```python
from build123d import *

# Parameters (mm, degrees)
F0_R     = 3.5
F0_W     = 5
F0_H     = 25
F1_DEPTH = 1
F2_W     = 2
F2_H     = 12
F2_H_2   = 8
F3_DEPTH = 9.5
F4_W     = 23
F4_H     = 35
F5_DEPTH = 1


with BuildPart() as f1:
    # F0 (on Top) → F1 (new body)
    with BuildSketch(Plane.XY):
        with BuildLine():
            Line((3.5, -20), (13.5, -20))
            Line((13.5, -20), (13.5, 10))
            Line((13.5, 10), (3.5, 20))
            Line((3.5, 20), (3.5, 28.319805))
            Line((3.5, 28.319805), (26.946408, 28.319805))
            ThreePointArc((26.946408, 28.319805), (30.556224, 25.954367), (34.819805, 26.623653))
            ThreePointArc((34.819805, 26.623653), (36.975362, 27.961046), (39.041812, 29.432384))
            ThreePointArc((39.041812, 29.432384), (40.225162, 31.819805), (39.041812, 34.207227))
            ThreePointArc((39.041812, 34.207227), (36.975362, 35.678564), (34.819805, 37.015958))
            ThreePointArc((34.819805, 37.015958), (30.556224, 37.685243), (26.946408, 35.319805))
            Line((26.946408, 35.319805), (-26.946408, 35.319805))
            ThreePointArc((-26.946408, 35.319805), (-30.556224, 37.685243), (-34.819805, 37.015958))
            ThreePointArc((-34.819805, 37.015958), (-36.975362, 35.678564), (-39.041812, 34.207227))
            ThreePointArc((-39.041812, 34.207227), (-40.225162, 31.819805), (-39.041812, 29.432384))
            ThreePointArc((-39.041812, 29.432384), (-36.975362, 27.961046), (-34.819805, 26.623653))
            ThreePointArc((-34.819805, 26.623653), (-30.556224, 25.954367), (-26.946408, 28.319805))
            Line((-26.946408, 28.319805), (-3.5, 28.319805))
            Line((-3.5, 28.319805), (-3.5, 20))
            Line((-3.5, 20), (-13.5, 10))
            Line((-13.5, 10), (-13.5, -20))
            Line((-13.5, -20), (-3.5, -20))
            Line((-3.5, -20), (-3.5, -28.319805))
            Line((-3.5, -28.319805), (-26.946408, -28.319805))
            ThreePointArc((-26.946408, -28.319805), (-30.556224, -25.954367), (-34.819805, -26.623653))
            ThreePointArc((-34.819805, -26.623653), (-36.975362, -27.961046), (-39.041812, -29.432384))
            ThreePointArc((-39.041812, -29.432384), (-40.225162, -31.819805), (-39.041812, -34.207227))
            ThreePointArc((-39.041812, -34.207227), (-36.975362, -35.678564), (-34.819805, -37.015958))
            ThreePointArc((-34.819805, -37.015958), (-30.556224, -37.685243), (-26.946408, -35.319805))
            Line((-26.946408, -35.319805), (26.946408, -35.319805))
            ThreePointArc((26.946408, -35.319805), (30.556224, -37.685243), (34.819805, -37.015958))
            ThreePointArc((34.819805, -37.015958), (36.975362, -35.678564), (39.041812, -34.207227))
            ThreePointArc((39.041812, -34.207227), (40.225162, -31.819805), (39.041812, -29.432384))
            ThreePointArc((39.041812, -29.432384), (36.975362, -27.961046), (34.819805, -26.623653))
            ThreePointArc((34.819805, -26.623653), (30.556224, -25.954367), (26.946408, -28.319805))
            Line((26.946408, -28.319805), (3.5, -28.319805))
            Line((3.5, -28.319805), (3.5, -20))
        make_face()
        with Locations((-31.819805, -31.819805)):
            Circle(F0_R, mode=Mode.SUBTRACT)
        with Locations((31.819805, -31.819805)):
            Circle(F0_R, mode=Mode.SUBTRACT)
        with Locations((-4, 0)):
            Rectangle(F0_W, F0_H, mode=Mode.SUBTRACT)
        with Locations((-31.819805, 31.819805)):
            Circle(F0_R, mode=Mode.SUBTRACT)
        with Locations((4, 0)):
            Rectangle(F0_W, F0_H, mode=Mode.SUBTRACT)
        with Locations((31.819805, 31.819805)):
            Circle(F0_R, mode=Mode.SUBTRACT)
    extrude(amount=F1_DEPTH)

    # F2 (on face) → F3 (join)
    with BuildSketch(Plane.XY.offset(1)):
        with Locations((-10.5, 3)):
            Rectangle(F2_W, F2_H)
        with Locations((10.5, 3)):
            Rectangle(F2_W, F2_H)
        with Locations((10.5, -9)):
            Rectangle(F2_W, F2_H_2)
    extrude(amount=F3_DEPTH)

    # F4 (on face) → F5 (join)
    with BuildSketch(Plane.XY.offset(10.5)):
        Rectangle(F4_W, F4_H)
    extrude(amount=F5_DEPTH)


solid = f1.part
```
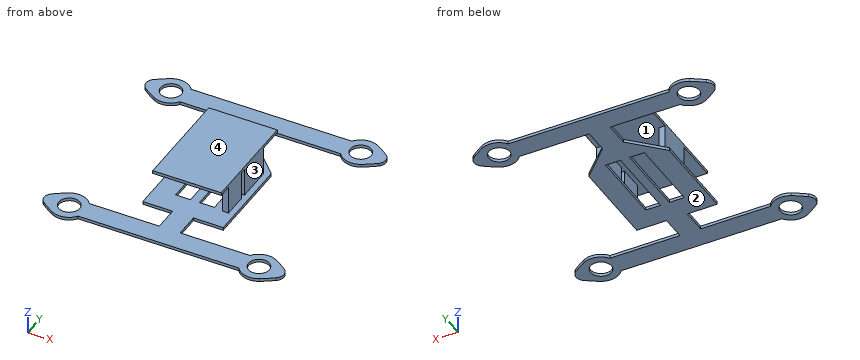
Here's how the part is built. I have some questions about the finished solid (model axes, mm). Face numbers are marked on the shaded views. Coordinates: 2 decimals unless noted, no trailing zeros. Loops run counter-clockwise (first coordinate to the right, second up) from the corner with the lowest first, then second, coordinate; pieces in that order, holes last. Notation, with made-up numbers: (-11.75, -27.75) - (42.25, -27.75) arc R15 ccw to (42.25, -1.75) - close; hole circle Ø11 at (17, 30). An arc over 180 degrees is marked (long way). Return JSON: item names as keys, results as strings. Group by question number.
Item 1: If we section it at B-B on y = -8: Write out the boundary of the cut face in (x, z).
Item 2: If we section it at C-C on z = 2.25: Write out the boundary of the cut face in (x, y).
Item 3: If we section it at A-A on x = -10.5: Write out the boundary of the cut face in (y, z).
Item 4: I need wall thicknesses on line 1 (X direction, y = 3.5, z = 6); line 2 (Z direction, x = -5, y = -13); line 3 (Z direction, x = -27.5, y = 28). Which ranges of each line are inside material? Lowest first, please. Write a range as from..to.
Item 5: If we section it at D-D on y = 14: Write out the boundary of the cut face in (x, z), and give its area (3 significant figures).
Item 6: Will these pins go through, and if not, where does the flat tip stop? P1, Ø0.8, axis at x = -10, z = 0.5, coming from the -Y side; P2, Ø8, axis at x = 31.82, y = -31.82, coming from the -Z side; P3, Ø1.5, axis at y = 12.5, z = 1.5, coming from the -X side; P4, Ø1.1, axis at x = -3, z = 11, coming from the -Y side.
Item 7: We'd pull the mould along Z, two halves only. Please class the marked faces 1, 2, 3 and 4: +Z half, -Z half, draft (parallel to the pull), parting line (faces both ways), or undercut.
Calculated:
{
 "1": {"outline": "(-13.5, 0) - (-6.5, 0) - (-6.5, 1) - (-13.5, 1) - close; (-11.5, 10.5) - (9.5, 10.5) - (9.5, 1) - (6.5, 1) - (6.5, 0) - (13.5, 0) - (13.5, 1) - (11.5, 1) - (11.5, 11.5) - (-11.5, 11.5) - close; (-1.5, 0) - (1.5, 0) - (1.5, 1) - (-1.5, 1) - close"},
 "2": {"outline": "(-11.5, -3) - (-9.5, -3) - (-9.5, 9) - (-11.5, 9) - close; (9.5, -13) - (11.5, -13) - (11.5, -5) - (9.5, -5) - close; (9.5, -3) - (11.5, -3) - (11.5, 9) - (9.5, 9) - close"},
 "3": {"outline": "(-35.32, 0) - (-28.32, 0) - (-28.32, 1) - (-35.32, 1) - close; (-20, 0) - (13, 0) - (13, 1) - (9, 1) - (9, 10.5) - (17.5, 10.5) - (17.5, 11.5) - (-17.5, 11.5) - (-17.5, 10.5) - (-3, 10.5) - (-3, 1) - (-20, 1) - close; (28.32, 0) - (35.32, 0) - (35.32, 1) - (28.32, 1) - close"},
 "4": {"line 1": "x = -11.5..-9.5, 9.5..11.5", "line 2": "z = 0..1, 10.5..11.5", "line 3": "z = 0..1"},
 "5": {"outline": "(-11.5, 10.5) - (11.5, 10.5) - (11.5, 11.5) - (-11.5, 11.5) - close; (-9.5, 0) - (9.5, 0) - (9.5, 1) - (-9.5, 1) - close", "area": "42.0 mm^2"},
 "6": {"P1": "stops at y = -35.32", "P2": "stops at z = 0", "P3": "stops at x = -11.56", "P4": "stops at y = -17.5"},
 "7": {"face 1": "undercut", "face 2": "-Z half", "face 3": "draft", "face 4": "+Z half"}
}
